```python
from build123d import *

# Parameters (mm, degrees)
SKETCH_R     = 100
PAD_DEPTH    = 2.5
SKETCH001_R  = 39.634074
PAD001_DEPTH = 60
SKETCH002_R  = 100
PAD002_DEPTH = 2.5
SKETCH003_R  = 28.45255
POCKET_DEPTH = 65.001


with BuildPart() as part:
    # Sketch → Pad (new body)
    with BuildSketch(Plane.XZ):
        Circle(SKETCH_R)
    extrude(amount=PAD_DEPTH)

    # Sketch001 → Pad001 (new body)
    with BuildSketch(Plane.XZ.offset(2.5)):
        Circle(SKETCH001_R)
    extrude(amount=PAD001_DEPTH)

    # Sketch002 → Pad002 (new body)
    with BuildSketch(Plane.XZ.offset(62.5)):
        Circle(SKETCH002_R)
    extrude(amount=PAD002_DEPTH)

    # Sketch003 → Pocket (cut, through all)
    with BuildSketch(Plane.XZ.offset(65)):
        Circle(SKETCH003_R)
    extrude(amount=-POCKET_DEPTH, mode=Mode.SUBTRACT)


solid = part.part
```
Work out the finished part from the listing and answer in its coordinate system (mm). A direction names the side the tool comes from. Give positions to 0.01 mm unless a question says otherwise; leave off trailing zeros. Write each loop counter-clockwise with the first axis right and the second up, starting at its lowest first coordinate (ties: lowest second). Pieces come first, ordered by that corner, then holes. Notation, with made-up numbers: (-18, -5.5) -> (31, -5.5) arc R28 ccw to (31, 24.5) -> close; hole circle Ø1 at (-27, 16). An arc over 180 degrees is marked (long way). Write item = value, one per line.
Q1. A tool of negligible diameter and unlimited length cuts with its end or side. For faces 1 (the cylindrical face through (95.38, -63.73, 30.04)), 2 (the flat face through (-1, -2.5, -43)), from which of +Z, -Z, +X, -X, +Y, -Y can it reach the whole face along a straight path? Write none if from no direction.
Computed values:
face_1 = +Y, -Y
face_2 = none
Q2. For a pull along Y with two mould halves and no side action, classify faces 3 (the cylindrical face through (-5.16, -32.08, 39.297)), 4 (the cylindrical face through (-6.168, -32.955, -27.776)), 5 (the flat face through (21, -65, -21)) as pulls with the +Y half, pulls with the -Y half, needs draft (parallel to the pull), parting line crosses it, or undercut.
Computed values:
face_3 = undercut
face_4 = needs draft
face_5 = pulls with the -Y half
Q3. Consider line 1 along Y through (x, z) = (34, -56); line 2 along Z through (x, y) = (0, -19); line 3 along Z through (x, y) = (-20, -46.5). Determine where each line is inside the solid, lowest interval first.
Computed values:
line_1 = -65 to -62.5, -2.5 to 0
line_2 = -39.63 to -28.45, 28.45 to 39.63
line_3 = -34.22 to -20.24, 20.24 to 34.22
Q4. Section D-D on z = 32 is taken. Determine the outline of the cut face in (x, y).
Computed values:
outline = (-94.74, -65) -> (94.74, -65) -> (94.74, -62.5) -> (23.39, -62.5) -> (23.39, -2.5) -> (94.74, -2.5) -> (94.74, 0) -> (-94.74, 0) -> (-94.74, -2.5) -> (-23.39, -2.5) -> (-23.39, -62.5) -> (-94.74, -62.5) -> close
Q5. Section C-C on y = -36 is taken. Determine the outline of the cut face in (x, z).
Computed values:
outline = circle Ø79.27 at (0, 0); hole circle Ø56.91 at (0, 0)
Q6. Section B-B on z = 0 is taken. Determine the outline of the cut face in (x, y), and give its area (3 significant figures).
Computed values:
outline = (-100, -65) -> (-28.45, -65) -> (-28.45, 0) -> (-100, 0) -> (-100, -2.5) -> (-39.63, -2.5) -> (-39.63, -62.5) -> (-100, -62.5) -> close; (28.45, -65) -> (100, -65) -> (100, -62.5) -> (39.63, -62.5) -> (39.63, -2.5) -> (100, -2.5) -> (100, 0) -> (28.45, 0) -> close
area = 2,060 mm^2
Q7. Section A-A on x = 0 is taken. Determine the outline of the cut face in (y, z), and give its area (3 significant figures).
Computed values:
outline = (-65, -100) -> (-62.5, -100) -> (-62.5, -39.63) -> (-2.5, -39.63) -> (-2.5, -100) -> (0, -100) -> (0, -28.45) -> (-65, -28.45) -> close; (-65, 28.45) -> (0, 28.45) -> (0, 100) -> (-2.5, 100) -> (-2.5, 39.63) -> (-62.5, 39.63) -> (-62.5, 100) -> (-65, 100) -> close
area = 2,060 mm^2
Q8. Flat-ended cylindrical pins translate along their axes: pin 1 Ø1 at (y, z) = (-17.5, -10) entering from -X; pin 2 Ø2 at (y, z) = (-34, -18) entering from -X; pin 3 Ø12 at (x, y) = (-79, -55) entering from +Z; pin 4 Ø4 at (x, y) = (-36.5, -13.5) entering from +Z. Find the tip coordinate at first contact, or state that the pin passes through.
Computed values:
pin_1 = -38.48
pin_2 = -35.8
pin_3 = through
pin_4 = 19.51
